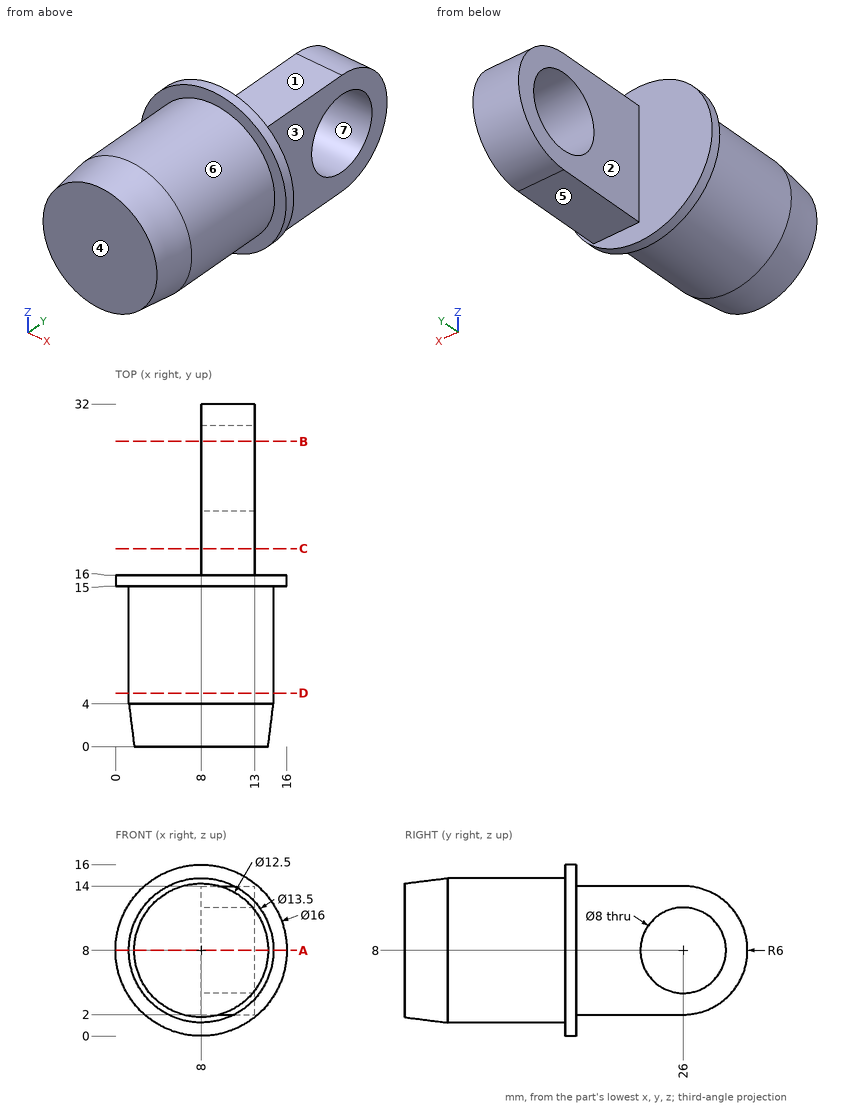
Geometry: see drawing. Coordinates: mm, zero at the bounding-box minimum. A direction names the side the tool comes from. Coordinates: 2 decimals unless noted, no trailing zeros. Order: outer loops, then holes, each group sorted by start corner. A loop starts at its lowest first (then second) coordinate and runs counter-clockwise, first axis right, second up. Notation, with made-up numbers: M 41.5,87.25 L 97.5,87.25 A14 ccw 97.5,103.25 Z; hole C 58.25,-14.75 d7. An arc over 180 degrees is marked long. Write item = value, one per line. Start each with the question number.
(1) Section C-C on y = 18.5. Output: boundary loops of the cut face in (x, z), and give its area (3 significant figures).
(2) Pull-direction query (Z, two-part tool) for the marked faces 5, 6 and 7; classes: released by +Z, released by -Z, zero draft, split by the parting line, or undercut.
(3) First-contact query: P1, Ø5.5, axis at x = 9.5, y = 21, coming from the -Z side; P2, Ø6, axis at y = 27, z = 7.5, coming from the -X side; P3, Ø6, axis at x = 4, y = 5, coming from the -Z side. Flat tips, straight axial feed; report the tip coordinate or a pass-through.
(4) Line query: line 1 along Z through (x, y) = (11.85, 26); line 2 along Y through (x, z) = (6, 5.25); line 3 along Z through (x, y) = (9.25, 28.5). Output: solid intervals per line, ascending. Write a range as [from, to].
(5) Section B-B on y = 28.5. Output: boundary loops of the cut face in (x, z).
(6) Section A-A on z = 8. Output: boundary loops of the cut face in (x, y), and give its area (4 significant figures).
(7) Section D-D on y = 5. Output: boundary loops of the cut face in (x, z).
(8) Reachability of the marked faces 1, 2, 3 and 4 from +Z, -Z, +X, -X, +Y, -Y: full face, straight path, thin tool, end or side. Return the list, or none.
Result set:
q1.outline = M 8,2 L 13,2 L 13,14 L 8,14 Z
q1.area = 60.0 mm²
q2.face_5 = released by -Z
q2.face_6 = split by the parting line
q2.face_7 = undercut
q3.P1 = 2
q3.P2 = 8
q3.P3 = 1.32
q4.line_1 = [2, 4], [12, 14]
q4.line_2 = [0, 16]
q4.line_3 = [2.55, 4.88], [11.12, 13.45]
q5.outline = M 8,2.55 L 13,2.55 L 13,4.88 L 8,4.88 Z; M 8,11.12 L 13,11.12 L 13,13.45 L 8,13.45 Z
q6.outline = M 0,15 L 1.25,15 L 1.25,4 L 1.75,0 L 14.25,0 L 14.75,4 L 14.75,15 L 16,15 L 16,16 L 13,16 L 13,22 L 8,22 L 8,16 L 0,16 Z; M 8,30 L 13,30 L 13,32 L 8,32 Z
q6.area = 256.5 mm²
q7.outline = C 8,8 d13.5
q8.face_1 = +Z, +X, -X, +Y
q8.face_2 = +Z, -Z, -X, +Y
q8.face_3 = +Z, -Z, +X, +Y
q8.face_4 = +Z, -Z, +X, -X, -Y
